from build123d import *

# Parameters (mm, degrees)
F4_W         = 39.45
F4_H         = 6.43
F4_W_2       = 26.5
F4_R         = 2.105
F4_R_2       = 2.05
F5_DEPTH     = 1.6
F7_DEPTH     = 3.1
F6_W         = 5
F6_H         = 22.5
F8_DEPTH     = 8.5
F9_R         = 1
F10_W        = 21.6
F10_H        = 1.4
F11_DEPTH    = 3.1
F12_T1_DEPTH = 21.6
F13_W        = 21.6
F13_H        = 1.4
F14_DEPTH    = 3.1
F15_T1_DEPTH = 21.6


# Not quite as in the source:
# - a fillet or chamfer that OpenCascade refuses, or shapes differently, is made with other operations: its cross-section is extruded or revolved along the edge and cut away or added
# - a feature names something its author has since deleted; it is built from what else it names


with BuildPart() as f5:
    # F4 (on Top) → F5 (new body)
    with BuildSketch(Plane.XY):
        with Locations((2.695, -15.585)):
            Rectangle(F4_W, F4_H)
        with Locations((37.87, -15.585)):
            Rectangle(F4_W_2, F4_H)
        Polygon((85, 12.23), (-27, 12.23), (-27, -12.37), (-17.03, -12.37), (22.42, -12.37), (24.62, -12.37), (51.12, -12.37), (85, -12.37), align=None)
        Circle(F4_R, mode=Mode.SUBTRACT)
        with Locations((28.1, 0)):
            Circle(F4_R_2, mode=Mode.SUBTRACT)
        with Locations((46.1, 0)):
            Circle(F4_R_2, mode=Mode.SUBTRACT)
        with Locations((57, 0)):
            Circle(F4_R, mode=Mode.SUBTRACT)
        with Locations((66.1, 0)):
            Circle(F4_R_2, mode=Mode.SUBTRACT)
    extrude(amount=F5_DEPTH)

    # F6 (on face) → F7 (join)
    with BuildSketch(Plane.XY.offset(1.6)):
        Polygon((-9.65, 11.25), (-14.65, 11.25), (-14.65, -11.25), (-9.65, -11.25), (-9.65, 0), align=None)
    extrude(amount=F7_DEPTH)

    # F6 (on face) → F8 (join)
    with BuildSketch(Plane.XY.offset(1.6)):
        with Locations((-21.05, 0)):
            Rectangle(F6_W, F6_H)
    extrude(amount=F8_DEPTH)

    # F9
    f9_edges = [f5.edges().sort_by_distance(p)[0] for p in [
        (-27, -12.37, 0.8),
        (-17.03, -12.37, 0.8),
        (-17.03, -18.8, 0.8),
        (24.62, -12.37, 0.8),
        (24.62, -18.8, 0.8),
        (22.42, -18.8, 0.8),
        (51.12, -18.8, 0.8),
        (22.42, -12.37, 0.8),
        (51.12, -12.37, 0.8),
        (85, 12.23, 0.8),
        (-27, 12.23, 0.8),
        (85, -12.37, 0.8),
    ]]
    fillet(f9_edges, radius=F9_R)

    # F10 (on face) → F11 (cut)
    with BuildSketch(Plane.YZ.offset(-9.65)):
        with Locations((0, 3.84)):
            Rectangle(F10_W, F10_H)
    extrude(amount=-F11_DEPTH, mode=Mode.SUBTRACT)

    # F12: fillet of radius 2 on 1 edges, made by hand

    # F12_s2 → F12_t1 (join)
    with BuildSketch(Plane.XZ.offset(-10.8)):
        with BuildLine():
            ThreePointArc((-10.8421215972, 4.54), (-12.0253375538, 4.1524515497), (-12.75, 3.14))
            Line((-12.75, 3.14), (-12.75, 4.54))
            Line((-12.75, 4.54), (-10.8421215972, 4.54))
        make_face()
    extrude(amount=F12_T1_DEPTH)

    # F13 (on face) → F14 (cut)
    with BuildSketch(Plane.YZ.offset(-18.55)):
        with Locations((0, 8.95)):
            Rectangle(F13_W, F13_H)
    extrude(amount=-F14_DEPTH, mode=Mode.SUBTRACT)

    # F15: fillet of radius 2 on 1 edges, made by hand

    # F15_s2 → F15_t1 (join)
    with BuildSketch(Plane.XZ.offset(-10.8)):
        with BuildLine():
            ThreePointArc((-19.7421215972, 9.65), (-20.9253375538, 9.2624515497), (-21.65, 8.25))
            Line((-21.65, 8.25), (-21.65, 9.65))
            Line((-21.65, 9.65), (-19.7421215972, 9.65))
        make_face()
    extrude(amount=F15_T1_DEPTH)


solid = f5.part
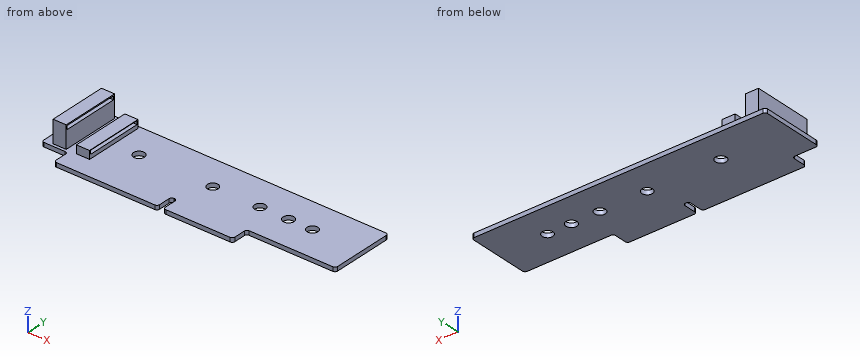
Work out the finished part from the listing and answer in its coordinate system (mm). Give positions to 0.01 mm unless a question says otherwise; leave off trailing zeros. Loops run counter-clockwise (first coordinate to the right, second up) from the corner with the lowest first, then second, coordinate; pieces in that order, holes last. Notation, with made-up numbers: (-29.75, 38) -> (7.25, 38) arc R17 ccw to (7.25, 66) -> close; hole circle Ø9 at (68, 8). An arc over 180 degrees is marked (long way). Use a Markdown table: item, result. Add a question column.
1) Each of these flat-tipped pins is pushed along its axis until it touches: P1, Ø4, axis at y = -4.5, z = 8.5, coming from the -X side; P2, Ø1.6, axis at x = -11.5, z = 3, coming from the -Y side; P3, Ø1.5, axis at x = -11, y = -4.5, coming from the +Z side. Where does it stop, or does it pass through?
2) The part is cut by section D-D, the plane y = -8. Determine the outline of the cut face in (x, z), plus the area to 3 significant figures.
3) Consider line 1 along Y through (x, z) = (66.1, 0.95); line 2 along X through (y, z) = (-8.5, 1.75); line 3 along Y through (x, z) = (28.1, 1.25). Determine where each line is inside the solid, lowest interval first.
4) The part is cut by section C-C, the plane x = 0. Determine the outline of the cut face in (y, z) (3 decimals), plus the area to 3 significant figures.
5) The part is cut by section A-A, the plane x = 57. Determine the outline of the cut face in (y, z) (3 decimals), plus the area to 3 significant figures.
6) The part is cut by section B-B, the plane y = 0. Count the separate pieces of the cut face and the enclosed holes in it, plus the area to 3 significant figures.
Reported:
| question | item | result |
|---|---|---|
| 1 | P1 | stops at x = -23.55 |
| 1 | P2 | stops at y = -11.25 |
| 1 | P3 | stops at z = 4.7 |
| 2 | outline | (-27, 0) -> (85, 0) -> (85, 1.6) -> (-9.65, 1.6) -> (-9.65, 3.14) -> (-12.75, 3.14) arc R2 cw to (-10.84, 4.54) -> (-9.65, 4.54) -> (-9.65, 4.7) -> (-14.65, 4.7) -> (-14.65, 1.6) -> (-18.55, 1.6) -> (-18.55, 8.25) -> (-21.65, 8.25) arc R2 cw to (-19.74, 9.65) -> (-18.55, 9.65) -> (-18.55, 10.1) -> (-23.55, 10.1) -> (-23.55, 1.6) -> (-27, 1.6) -> close |
| 2 | area | 230 mm^2 |
| 3 | line 1 | y = -12.37 to -2.05, 2.05 to 12.23 |
| 3 | line 2 | x = -23.55 to -18.55, -14.65 to -9.65 |
| 3 | line 3 | y = -18.8 to -2.05, 2.05 to 12.23 |
| 4 | outline | (-18.8, 0) -> (-2.105, 0) -> (-2.105, 1.6) -> (-18.8, 1.6) -> close; (2.105, 0) -> (12.23, 0) -> (12.23, 1.6) -> (2.105, 1.6) -> close |
| 4 | area | 42.9 mm^2 |
| 5 | outline | (-12.37, 0) -> (-2.105, 0) -> (-2.105, 1.6) -> (-12.37, 1.6) -> close; (2.105, 0) -> (12.23, 0) -> (12.23, 1.6) -> (2.105, 1.6) -> close |
| 5 | area | 32.6 mm^2 |
| 6 | separate pieces | 6 |
| 6 | enclosed holes | 0 |
| 6 | area | 197 mm^2 |
